Input: part model. Units: mm. Frame: model coordinates. A direction names the side the tool comes from. Coordinates: 2 decimals unless noted, no trailing zeros. Loops run counter-clockwise (first coordinate to the right, second up) from the corner with the lowest first, then second, coordinate; pieces in that order, holes last.
Item 1: Section D-D on x = -8.5. Return loops of the section in (y, z).
Item 2: Reachability of faces 1 (the flat face through (-6, 6, 30)), 2 (the flat face through (0, -12.5, 40)) from +Z, -Z, +X, -X, +Y, -Y: full face, straight path, thin tool, end or side. Return the list, or none.
Item 3: Ray query, line 1 along Z through (x, y) = (-10.5, 6); line 2 along X through (y, z) = (-1, 27.5); line 3 along X through (y, z) = (-7.25, 11). Return the intervals inside material, ascending.
Item 4: Section C-C on z = 23. Return loops of the section in (x, y).
Item 5: Contact query for flat-ended pins moving along their axis: P1, Ø5, axis at x = -9, y = 9.5, coming from the -Z side; P2, Ø5, axis at x = 7, z = 7.5, coming from the -Y side; P3, Ø3, axis at x = 8, z = 20, coming from the -Y side. Output: stop coordinate, or through.
Item 6: Section A-A on y = 0. Return loops of the section in (x, z).
Autodesk Inventor part; units mm, degrees
ref_plane "YZ Plane" through (0, 0, 0) normal (1, 0, 0) x (0, 1, 0)
ref_plane "XZ Plane" through (0, 0, 0) normal (0, 1, 0) x (-1, 0, 0)
ref_plane "XY Plane" through (0, 0, 0) normal (0, 0, 1) x (1, 0, 0)
sketch "Sketch1" plane through (0, 0, 0) normal (0, 1, 0) x (-1, 0, 0)
  line L0 (1.2262, 1.2262) -> (8, 8)
  line L1 (8, 8) -> (8, 50)
  line L2 (8, 50) -> (0, 50)
  line L3 (0, 50) -> (0, 1.2262)
  line L4 (0, 1.2262) -> (1.2262, 1.2262)
  point P0 (0, 0)
  dimension "d0" = 50
  dimension "d1" = 8
  dimension "d2" = 135
revolve "Revolution1" add sketch "Sketch1" angle 360 about axis through (0, 0, 50) along (0, 0, -1)
sketch "Sketch2" plane through (0, 0, 50) normal (0, 0, 1) x (1, 0, 0)
  circle A0 centre (0, 0) radius 8
  line L0 (-12.5, -12.5) -> (12.5, -12.5)
  line L1 (12.5, -12.5) -> (12.5, 12.5)
  line L2 (12.5, 12.5) -> (-12.5, 12.5)
  line L3 (-12.5, 12.5) -> (-12.5, -12.5)
  line L4 (-12.5, -12.5) -> (12.5, 12.5) construction
  line L5 (12.5, -12.5) -> (-12.5, 12.5) construction
  dimension "d4" = 25
  dimension "d6" = 25
extrude "Extrusion1" add sketch "Sketch2" against normal blind 20
properties part number "effector"
Results found:
1. outline: (-12.5, 30) - (12.5, 30) - (12.5, 50) - (-12.5, 50) - close
2. face 1: -Z
2. face 2: +Z, -Z, +X, -X, -Y
3. line 1: z = 30 to 50
3. line 2: x = -7.94 to 7.94
3. line 3: x = -3.38 to 3.38
4. outline: circle Ø16 at (0, 0)
5. P1: stops at z = 30
5. P2: stops at y = -6.58
5. P3: stops at y = -4.66
6. outline: (-12.5, 30) - (-8, 30) - (-8, 8) - (-1.23, 1.23) - (1.23, 1.23) - (8, 8) - (8, 30) - (12.5, 30) - (12.5, 50) - (-12.5, 50) - close
